Check sheet for the modelled part. Datum: model origin and axes. Units: mm. Give positions to 0.01 mm unless a question says otherwise; leave off trailing zeros. Loops run counter-clockwise (first coordinate to the right, second up) from the corner with the lowest first, then second, coordinate; pieces in that order, holes last.
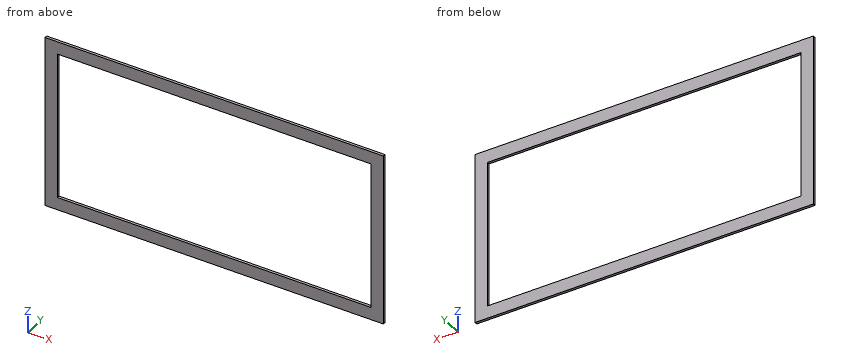
```python
from build123d import *

# Parameters (mm, degrees)
F1_DEPTH = 19.05


with BuildPart() as f1:
    # F0 (on Front) → F1 (new body)
    with BuildSketch(Plane.XZ):
        Polygon((1130.3, 520.7), (1219.2, 609.6), (-1219.2, 609.6), (-1130.3, 520.7), align=None)
        Polygon((1219.2, -609.6), (1219.2, 609.6), (1130.3, 520.7), (1130.3, -520.7), align=None)
        Polygon((-1219.2, -609.6), (1219.2, -609.6), (1130.3, -520.7), (-1130.3, -520.7), align=None)
        Polygon((-1130.3, 520.7), (-1219.2, 609.6), (-1219.2, -609.6), (-1130.3, -520.7), align=None)
    extrude(amount=F1_DEPTH)


solid = f1.part
```
(1) Section check A-A on x = 309. Record the boundary of the cut face in (y, z), plus the area to 3 significant figures.
(2) Material ranges on line 1 (X direction, y = -1, z = 334); line 2 (Z direction, x = -1105.5, y = -17), recorded low to high.
(3) Section check B-B on z = 341. Record the boundary of the cut face in (x, y).
(4) Section check C-C on y = -4.75. Record the boundary of the cut face in (x, z).
Computed values:
1. outline: (-19.05, -609.6) - (0, -609.6) - (0, -520.7) - (-19.05, -520.7) - close; (-19.05, 520.7) - (0, 520.7) - (0, 609.6) - (-19.05, 609.6) - close
1. area: 3,390 mm2
2. line 1: x = -1219.2 to -1130.3, 1130.3 to 1219.2
2. line 2: z = -609.6 to -520.7, 520.7 to 609.6
3. outline: (-1219.2, -19.05) - (-1130.3, -19.05) - (-1130.3, 0) - (-1219.2, 0) - close; (1130.3, -19.05) - (1219.2, -19.05) - (1219.2, 0) - (1130.3, 0) - close
4. outline: (-1219.2, -609.6) - (1219.2, -609.6) - (1219.2, 609.6) - (-1219.2, 609.6) - close; hole (-1130.3, -520.7) - (1130.3, -520.7) - (1130.3, 520.7) - (-1130.3, 520.7) - close
